The model under review builds one solid part; all positions refer to its coordinate system, in mm. A direction names the side the tool comes from. Coordinates: 2 decimals unless noted, no trailing zeros. Loops run counter-clockwise (first coordinate to the right, second up) from the corner with the lowest first, then second, coordinate; pieces in that order, holes last. Notation, with made-up numbers: (73.5, 43) - (89.5, 43) arc R16 ccw to (89.5, 64) - close; hole circle Ø6 at (18.5, 43). An arc over 180 degrees is marked (long way). One line per item, written item: value. Start each with the question number.
1. Mouldability with a two-part tool opening along X and no side actions: class faces 1 (the face through (-1.73, 7.81, 22.53)), 2 (the face through (0, 0, 57.45)), 3 (the face through (6.583, 3.55, 40.77)) as +X half, -X half, draft (parallel to the pull), parting line (faces both ways), or undercut.
2. We need section A-A, the plane y = 0. Give the boundary of the cut face in (x, z), then the cut area to 3 significant figures.
3. To check wall thickness, follow line 1 (Y direction, x = 0, z = 38.5); line 2 (Z direction, x = 4.75, y = -5.5); line 3 (X direction, y = 6.25, z = 11). State the ranges of each line that lie inside material, in increasing order.
4. We need section D-D, the plane z = 51. Give the boundary of the cut face in (x, y), then the cut area to 3 significant figures.
5. For faces 4 (the face through (0, -1.3, 54)), 5 (the face through (-0.13, -5.51, 40.77)), 6 (the face through (0, 0, 0)), list the 3-axis set-ups (+Z, -Z, +X, -X, +Y, -Y) from which the entire face can be reached by the end or side of a thin tool; tool diameter is ignored.
6. We need section B-B, the plane x = 0. Give the boundary of the cut face in (y, z).
7. Insertion check: P1, Ø1, axis at y = 3, z = 28.5, coming from the -X side; P2, Ø2, axis at x = 5, y = 4, coming from the +Z side; P3, Ø8, axis at y = -6, z = 36.5, coming from the -X side; P4, Ø1, axis at x = -3, z = 51, coming from the +Y side. Each pin has a flat end and moves straight along its axis. Give the tip position at first contact, or say it passes through.
8. We need section C-C, the plane z = 42.5. Give the boundary of the cut face in (x, y), then the cut area to 3 significant figures.
Autodesk Inventor part; units mm, degrees
ref_plane "Work Plane5" through (0, -1.5, 46.8) normal (0, 1, 0) x (-1, 0, 0)
ref_plane "YZ Plane" through (0, 0, 0) normal (1, 0, 0) x (0, 1, 0)
ref_plane "XY Plane" through (0, 0, 0) normal (0, 0, 1) x (1, 0, 0)
sketch "Sketch1" plane through (0, 0, 0) normal (0, 0, 1) x (1, 0, 0)
  circle A0 centre (0, 0) radius 8
  dimension "d0" = 16
extrude "Extrusion1" add sketch "Sketch1" along normal blind 45.7
sketch "Sketch2" plane through (0, 0, 45.7) normal (0, 0, 1) x (1, 0, 0)
  line L0 (0, 0) -> (0, -6.5)
  circle A0 centre (0, -6.5) radius 1
  circle A1 centre (5.6292, 3.25) radius 1
  circle A2 centre (-5.6292, 3.25) radius 1
  dimension "d8" = 360
  dimension "d38" = 6.5
  dimension "d39" = 2
  dimension "d42" = 360
extrude "Extrusion2" cut sketch "Sketch2" against normal blind 10
sketch "Sketch3" plane through (0, 0, 45.7) normal (0, 0, 1) x (1, 0, 0)
  circle A0 centre (0, 0) radius 5
  dimension "d12" = 10
extrude "Extrusion3" add sketch "Sketch3" along normal blind 1.1
sketch "Sketch8" plane through (0, 0, 46.8) normal (0, 0, 1) x (1, 0, 0)
  circle A0 centre (0, 0) radius 1.5
  dimension "d31" = 3
extrude "Extrusion8" add sketch "Sketch8" along normal blind 10.65
ref_plane "Work Plane5" through (0, -1.5, 46.8) normal (0, 1, 0) x (-1, 0, 0)
sketch "Sketch9" plane through (0, -1.5, 46.8) normal (0, 1, 0) x (-1, 0, 0)
  line L0 (1.5, 10.65) -> (-1.5, 10.65)
  line L1 (0, 10.65) -> (1.5, 10.65)
  line L2 (1.5, 10.65) -> (1.5, 2.85)
  line L3 (1.5, 2.85) -> (-1.5, 2.85)
  line L4 (-1.5, 2.85) -> (-1.5, 10.65)
  line L5 (-1.5, 10.65) -> (0, 10.65)
  point P0 (0, -46.8)
  dimension "d34" = 1.5
  dimension "d35" = 7.8
extrude "Extrusion9" cut sketch "Sketch9" along normal blind 0.2
properties part number "Motor"
Findings below:
1. face 1: parting line
1. face 2: draft
1. face 3: undercut
2. outline: (-8, 0) - (8, 0) - (8, 45.7) - (5, 45.7) - (5, 46.8) - (1.5, 46.8) - (1.5, 57.45) - (-1.5, 57.45) - (-1.5, 46.8) - (-5, 46.8) - (-5, 45.7) - (-8, 45.7) - close
2. area: 774 mm2
3. line 1: -8 to -7.5, -5.5 to 8
3. line 2: 0 to 45.7
3. line 3: -4.99 to 4.99
4. outline: (-0.75, -1.3) - (0.75, -1.3) arc R1.5 ccw (long way) to start
4. area: 6.87 mm2
5. face 4: +Z, +X, -X, -Y
5. face 5: +Z
5. face 6: -Z, +X, -X, +Y, -Y
6. outline: (-8, 0) - (8, 0) - (8, 45.7) - (5, 45.7) - (5, 46.8) - (1.5, 46.8) - (1.5, 57.45) - (-1.3, 57.45) - (-1.3, 49.65) - (-1.5, 49.65) - (-1.5, 46.8) - (-5, 46.8) - (-5, 45.7) - (-5.5, 45.7) - (-5.5, 35.7) - (-7.5, 35.7) - (-7.5, 45.7) - (-8, 45.7) - close
7. P1: x = -7.6
7. P2: z = 45.7
7. P3: x = -7.75
7. P4: through
8. outline: circle Ø16 at (0, 0); hole circle Ø2 at (-5.63, 3.25); hole circle Ø2 at (0, -6.5); hole circle Ø2 at (5.63, 3.25)
8. area: 192 mm2
